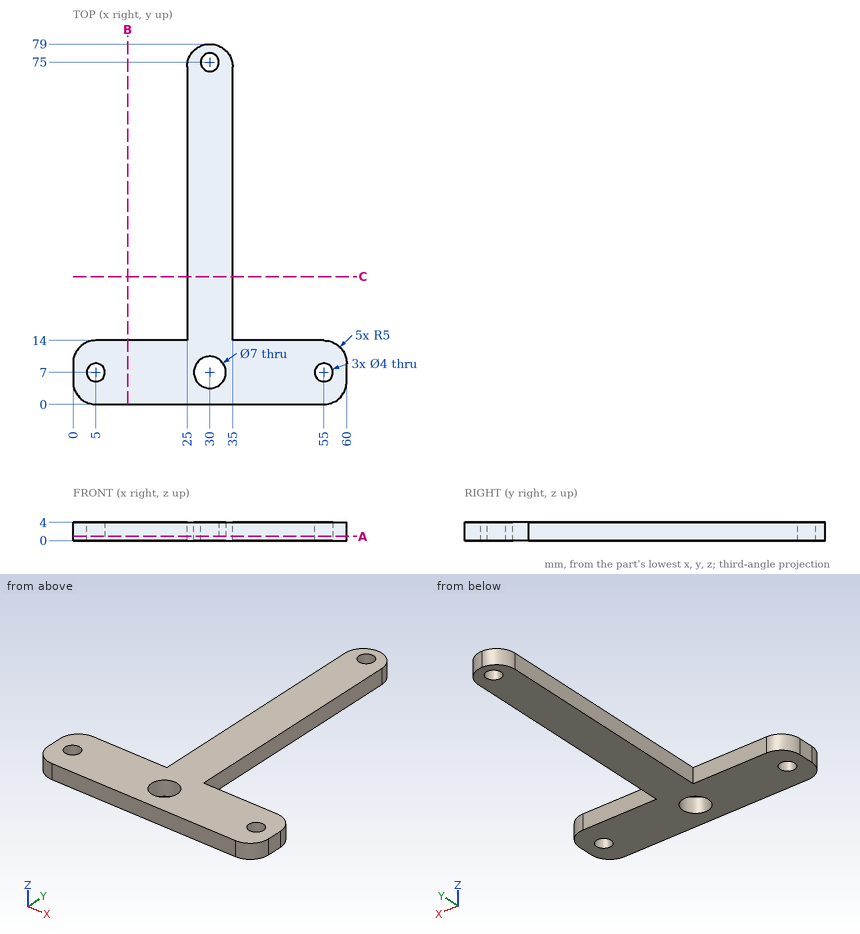
Verification items for this drawing (mm, ordinates from the low corner). Coordinates: 2 decimals unless noted, no trailing zeros. Order: outer loops, then holes, each group sorted by start corner. A loop starts at its lowest first (then second) coordinate and runs counter-clockwise, first axis right, second up. Notation, with made-up numbers: M 6.25,68.5 L 12.25,68.5 A8 cw 12.25,80.5 Z; hole C -1,81.25 d3. An arc over 180 degrees is marked long. One line per item, written item: value. Start each with the question number.
Item 1: Depth check by flat-ended pin: P1, Ø2, axis at y = 50, z = 3, coming from the -X side; P2, Ø3.5, axis at x = 5, y = 7, coming from the -Z side. Enter the tip coordinate at first touch or a pass-through.
Item 2: Thickness scan on probe 1 along Y at (x, z) = (30, 1.55); probe 2 along Y at (x, z) = (55, 1.15); probe 3 along X at (y, z) = (6, 3.05). Record the ranges inside material, lowest first.
Item 3: Sectioned sample at C-C on y = 28. Record the cut outline in (x, z), then the cut area to 3 significant figures.
Item 4: Sectioned sample at A-A on z = 0.9. Give the number of separate pieces and of enclosed holes in the cut face, then the cut area to 3 significant figures.
Item 5: Sectioned sample at B-B on x = 12. Record the cut outline in (y, z).
Calculated:
1. P1: x = 25
1. P2: through
2. probe 1: 0 to 3.5, 10.5 to 73, 77 to 79
2. probe 2: 0 to 5, 9 to 14
2. probe 3: 0 to 3.27, 6.73 to 26.65, 33.35 to 53.27, 56.73 to 60
3. outline: M 25,0 L 35,0 L 35,4 L 25,4 Z
3. area: 40.0 mm^2
4. separate pieces: 1
4. enclosed holes: 4
4. area: 1,380 mm^2
5. outline: M 0,0 L 14,0 L 14,4 L 0,4 Z
